For this review, take the finished solid that the model builds, in its own axes (mm). A direction names the side the tool comes from. Round coordinates to 2 decimals unless told otherwise and drop trailing zeros. Order: outer loops, then holes, each group sorted by start corner. A loop starts at its lowest first (then second) coordinate and runs counter-clockwise, first axis right, second up. Notation, with made-up numbers: (87.25, 64) - (93.25, 64) arc R13 cw to (93.25, 89) - close; hole circle Ø4 at (-20, 41). An arc over 180 degrees is marked (long way). One line per item, written item: value.
```python
from build123d import *

# Parameters (mm, degrees)
SKETCH1_W            = 609.6
SKETCH1_H            = 558.8
MAIN_BODY_DEPTH      = 6.35
SKETCH2_W            = 6.35
SKETCH2_H            = 152.4
CUT_EXTRUDE1_DEPTH   = 414.530799941
SKETCH8_W            = 127
SKETCH8_H            = 114.3
CUT_EXTRUDE5_DEPTH   = 414.530799941
FILLET3_R            = 12.7
FILLET3_OF_MIRROR3_R = 12.7
SKETCH9_W            = 88.9
SKETCH9_H            = 6.35
CUT_EXTRUDE7_DEPTH   = 414.530799941
SKETCH10_W           = 6.35
SKETCH10_H           = 25.4
CUT_EXTRUDE8_DEPTH   = 414.530799941
SKETCH11_W           = 12.7
SKETCH11_H           = 6.35
CUT_EXTRUDE9_DEPTH   = 414.530799941
SKETCH12_W           = 76.2
SKETCH12_H           = 6.35
CUT_EXTRUDE10_DEPTH  = 414.530799941


with BuildPart() as part:
    # Sketch1 → Main Body (new body)
    with BuildSketch(Plane(origin=(0, 0, 0), x_dir=(0, 0, -1), z_dir=(1, 0, 0))):
        Rectangle(SKETCH1_W, SKETCH1_H)
    extrude(amount=MAIN_BODY_DEPTH)

    # Sketch2 → Cut-Extrude1 (cut, through all)
    with BuildSketch(Plane(origin=(6.35, 0, 0), x_dir=(0, 0, -1), z_dir=(1, 0, 0))):
        with Locations((-200.025, 146.05)):
            Rectangle(SKETCH2_W, SKETCH2_H)
        with Locations((200.025, 146.05)):
            Rectangle(SKETCH2_W, SKETCH2_H)
    extrude(amount=-CUT_EXTRUDE1_DEPTH, mode=Mode.SUBTRACT)

    # Sketch8 → Cut-Extrude5 (cut, through all)
    with BuildSketch(Plane(origin=(6.35, 0, 0), x_dir=(0, 0, -1), z_dir=(1, 0, 0))):
        with Locations((-122.359674, 31.75)):
            Rectangle(SKETCH8_W, SKETCH8_H)
    cut_extrude5 = extrude(amount=-CUT_EXTRUDE5_DEPTH, mode=Mode.SUBTRACT)

    # Fillet3
    fillet3_edges = [part.edges().sort_by_distance(p)[0] for p in [
        (3.175, 88.9, 58.859674),
        (3.175, -25.4, 58.859674),
        (3.175, -25.4, 185.859674),
        (3.175, 88.9, 185.859674),
    ]]
    fillet(fillet3_edges, radius=FILLET3_R)

    # Mirror3: Cut-Extrude5 across plane
    add(cut_extrude5.mirror(Plane.XY), mode=Mode.SUBTRACT)

    # Fillet3 of Mirror3
    fillet3_of_mirror3_edges = [part.edges().sort_by_distance(p)[0] for p in [
        (3.175, 88.9, -58.859674),
        (3.175, -25.4, -58.859674),
        (3.175, -25.4, -185.859674),
        (3.175, 88.9, -185.859674),
    ]]
    fillet(fillet3_of_mirror3_edges, radius=FILLET3_OF_MIRROR3_R)

    # Sketch9 → Cut-Extrude7 (cut, through all)
    with BuildSketch(Plane(origin=(6.35, 0, 0), x_dir=(0, 0, -1), z_dir=(1, 0, 0))):
        with Locations((-88.9, -263.525)):
            Rectangle(SKETCH9_W, SKETCH9_H)
    cut_extrude7 = extrude(amount=-CUT_EXTRUDE7_DEPTH, mode=Mode.SUBTRACT)

    # Mirror4: Cut-Extrude7 across plane
    add(cut_extrude7.mirror(Plane.XY), mode=Mode.SUBTRACT)

    # Sketch10 → Cut-Extrude8 (cut, through all)
    with BuildSketch(Plane(origin=(6.35, 0, 0), x_dir=(0, 0, -1), z_dir=(1, 0, 0))):
        with Locations((-200.025, -196.85)):
            Rectangle(SKETCH10_W, SKETCH10_H)
        with Locations((200.025, -196.85)):
            Rectangle(SKETCH10_W, SKETCH10_H)
    extrude(amount=-CUT_EXTRUDE8_DEPTH, mode=Mode.SUBTRACT)

    # Sketch11 → Cut-Extrude9 (cut, through all)
    with BuildSketch(Plane(origin=(6.35, 0, 0), x_dir=(0, 0, -1), z_dir=(1, 0, 0))):
        with Locations((-209.55, 73.025)):
            Rectangle(SKETCH11_W, SKETCH11_H)
        with Locations((209.55, 73.025)):
            Rectangle(SKETCH11_W, SKETCH11_H)
    extrude(amount=-CUT_EXTRUDE9_DEPTH, mode=Mode.SUBTRACT)

    # Sketch12 → Cut-Extrude10 (cut, through all)
    with BuildSketch(Plane(origin=(6.35, 0, 0), x_dir=(0, 0, -1), z_dir=(1, 0, 0))):
        with Locations((0, 73.025)):
            Rectangle(SKETCH12_W, SKETCH12_H)
    extrude(amount=-CUT_EXTRUDE10_DEPTH, mode=Mode.SUBTRACT)


solid = part.part
```
Item 1: Take a section at C-C (x = 2.25). Count the separate pieces of the cut face and the enclosed holes in it, plus the area to 3 significant figures.
Returned:
separate pieces: 1
enclosed holes: 9
area: 308,000 mm^2
Item 2: Take a section at A-A (y = 5). Write out the cut boundary in (x, z), plus the area to 3 significant figures.
Returned:
outline: (0, -304.8) - (6.35, -304.8) - (6.35, -185.86) - (0, -185.86) - close; (0, -58.86) - (6.35, -58.86) - (6.35, 58.86) - (0, 58.86) - close; (0, 185.86) - (6.35, 185.86) - (6.35, 304.8) - (0, 304.8) - close
area: 2,260 mm^2
Item 3: Wall thickness on line 1 (Z direction, x = 3.75, y = 204.5); line 2 (Z direction, x = 5, y = 74); line 3 (Y direction, x = 5.25, z = -102.5): over which ranges is each line inside the solid? List them lowest first.
Returned:
line 1: -304.8 to -203.2, -196.85 to 196.85, 203.2 to 304.8
line 2: -304.8 to -215.9, -196.85 to -185.86, -58.86 to -38.1, 38.1 to 58.86, 185.86 to 196.85, 215.9 to 304.8
line 3: -279.4 to -266.7, -260.35 to -25.4, 88.9 to 279.4
Item 4: The part is to be moulded in two halves that separate along Z. For faces 1 (the flat face through (6.35, 4, 4)), 2 (the cylindrical face through (3.1, 85.3, -62.7)), say which applies: +Z half, -Z half, draft (parallel to the pull), parting line (faces both ways), or undercut.
Returned:
face 1: draft
face 2: undercut
Item 5: Take a section at B-B (z = -110). Write out the cut boundary in (x, y), plus the area to 3 significant figures.
Returned:
outline: (0, -279.4) - (6.35, -279.4) - (6.35, -266.7) - (0, -266.7) - close; (0, -260.35) - (6.35, -260.35) - (6.35, -25.4) - (0, -25.4) - close; (0, 88.9) - (6.35, 88.9) - (6.35, 279.4) - (0, 279.4) - close
area: 2,780 mm^2
Item 6: Machinability: for faces 3 (the cylindrical face through (3.13, -21.58, -182.24)), 4 (the flat face through (0, 4, 4)), which of the approach directions +Z, -Z, +X, -X, +Y, -Y give a long, thin tool a straight path to every point of the face, cutting with its end or side? Answer none if there is none.
Returned:
face 3: +X, -X
face 4: +Z, -Z, -X, +Y, -Y
